from build123d import *

# Parameters (mm, degrees)
SKETCH1_R           = 3.25
SKETCH1_R_2         = 2.38125
SKETCH1_R_3         = 1.5875
SKETCH1_W           = 4
SKETCH1_H           = 4
BOSS_EXTRUDE1_DEPTH = 4


with BuildPart() as part:
    # Sketch1 → Boss-Extrude1 (new body)
    with BuildSketch(Plane(origin=(0, 0, 0), x_dir=(1, 0, 0), z_dir=(0, 1, 0))):
        with BuildLine():
            Line((-50.8, 14), (-36.8, 14))
            ThreePointArc((-36.8, 14), (-35.385786438, 13.414213562), (-34.8, 12))
            Line((-34.8, 12), (-34.8, 7.914556152))
            ThreePointArc((-34.8, 7.914556152), (-34.214213562, 6.500342589), (-32.8, 5.914556152))
            Line((-32.8, 5.914556152), (50.8, 5.914556152))
            ThreePointArc((50.8, 5.914556152), (56.714556152, 0), (50.8, -5.914556152))
            Line((50.8, -5.914556152), (-32.8, -5.914556152))
            ThreePointArc((-32.8, -5.914556152), (-34.214213562, -6.500342589), (-34.8, -7.914556152))
            Line((-34.8, -7.914556152), (-34.8, -12))
            ThreePointArc((-34.8, -12), (-35.385786438, -13.414213562), (-36.8, -14))
            Line((-36.8, -14), (-50.8, -14))
            Line((-50.8, -14), (-52.8, -14))
            ThreePointArc((-52.8, -14), (-66.8, 0), (-52.8, 14))
            Line((-52.8, 14), (-50.8, 14))
        make_face()
        with Locations(Location((-50.8, 0, 0), (0, 0, 270))):
            Circle(SKETCH1_R, mode=Mode.SUBTRACT)
        with Locations(Location((38.8, 0, 0), (0, 0, 270))):
            Circle(SKETCH1_R_2, mode=Mode.SUBTRACT)
        with Locations(Location((26.1, 0, 0), (0, 0, 270))):
            Circle(SKETCH1_R_3, mode=Mode.SUBTRACT)
        with BuildLine():
            Line((-57.252349378, 8.220116331), (-54.247145558, 5.214912511))
            ThreePointArc((-54.247145558, 5.214912511), (-54.247145558, 3.447145558), (-56.014912511, 3.447145558))
            Line((-56.014912511, 3.447145558), (-59.020116331, 6.452349378))
            ThreePointArc((-59.020116331, 6.452349378), (-59.020116331, 8.220116331), (-57.252349378, 8.220116331))
        make_face(mode=Mode.SUBTRACT)
        with BuildLine():
            Line((-42.579883669, 6.452349378), (-45.585087489, 3.447145558))
            ThreePointArc((-45.585087489, 3.447145558), (-47.352854442, 3.447145558), (-47.352854442, 5.214912511))
            Line((-47.352854442, 5.214912511), (-44.347650622, 8.220116331))
            ThreePointArc((-44.347650622, 8.220116331), (-42.579883669, 8.220116331), (-42.579883669, 6.452349378))
        make_face(mode=Mode.SUBTRACT)
        with BuildLine():
            Line((-44.347650622, -8.220116331), (-47.352854442, -5.214912511))
            ThreePointArc((-47.352854442, -5.214912511), (-47.352854442, -3.447145558), (-45.585087489, -3.447145558))
            Line((-45.585087489, -3.447145558), (-42.579883669, -6.452349378))
            ThreePointArc((-42.579883669, -6.452349378), (-42.579883669, -8.220116331), (-44.347650622, -8.220116331))
        make_face(mode=Mode.SUBTRACT)
        with BuildLine():
            Line((-59.020116331, -6.452349378), (-56.014912511, -3.447145558))
            ThreePointArc((-56.014912511, -3.447145558), (-54.247145558, -3.447145558), (-54.247145558, -5.214912511))
            Line((-54.247145558, -5.214912511), (-57.252349378, -8.220116331))
            ThreePointArc((-57.252349378, -8.220116331), (-59.020116331, -8.220116331), (-59.020116331, -6.452349378))
        make_face(mode=Mode.SUBTRACT)
        with Locations((49.8, 0)):
            Rectangle(SKETCH1_W, SKETCH1_H, mode=Mode.SUBTRACT)
        with Locations((-9.2, 0)):
            Rectangle(SKETCH1_W, SKETCH1_H, mode=Mode.SUBTRACT)
    extrude(amount=BOSS_EXTRUDE1_DEPTH)


solid = part.part
Read the model definition and answer for the solid it produces. Units are mm, in the model's axes. A direction names the side the tool comes from. Round coordinates to 2 decimals unless told otherwise and drop trailing zeros. Write each loop counter-clockwise with the first axis right and the second up, starting at its lowest first coordinate (ties: lowest second). Pieces come first, ordered by that corner, then holes.
Q1. The mould has two halves that part along Z. Classify faces 6 (the face through (-57.5, 1.97, -4.93)), 7 (the face through (-34.23, 1.972, -6.516)), 8 (the face through (56.713, 1.972, -0.13)): released by +Z, released by -Z, zero draft, split by the parting line, or undercut.
Values:
face 6: undercut
face 7: released by -Z
face 8: split by the parting line
Q2. Find section B-B on z = 0. Determine the outline of the cut face in (x, y).
Values:
outline: (-66.8, 0) - (-54.05, 0) - (-54.05, 4) - (-66.8, 4) - close; (-47.55, 0) - (-11.2, 0) - (-11.2, 4) - (-47.55, 4) - close; (-7.2, 0) - (24.51, 0) - (24.51, 4) - (-7.2, 4) - close; (27.69, 0) - (36.42, 0) - (36.42, 4) - (27.69, 4) - close; (41.18, 0) - (47.8, 0) - (47.8, 4) - (41.18, 4) - close; (51.8, 0) - (56.71, 0) - (56.71, 4) - (51.8, 4) - close
Q3. Find section D-D on y = 2.4. State how many separate pieces and enclosed holes the cut face has, and give its area (3 significant figures).
Values:
separate pieces: 1
enclosed holes: 9
area: 1,730 mm2
Q4. Straight lines are drawn through the part: line 1 (X direction, y = 2.35, z = 0); line 2 (Z direction, x = 51, y = 0.8); line 3 (X direction, y = 2.2, z = -0.75). For each, find the intervals that lie inside material, in ascending order.
Values:
line 1: x = -66.8 to -54.05, -47.55 to -11.2, -7.2 to 24.51, 27.69 to 36.42, 41.18 to 47.8, 51.8 to 56.71
line 2: z = -5.91 to -2, 2 to 5.91
line 3: x = -66.78 to -53.96, -47.64 to -11.2, -7.2 to 24.7, 27.5 to 36.54, 41.06 to 47.8, 51.8 to 56.67
Q5. Flat-ended cylindrical pins translate along their axes: P1, Ø1.2, axis at x = 14.5, y = 1.5, coming from the -Z side; P2, Ø2, axis at y = 1, z = -7.5, coming from the +X side; P3, Ø1.2, axis at x = 3.5, y = 3, coming from the +Z side. Find the tip coordinate at first contact, or state that the pin passes through.
Values:
P1: stops at z = -5.91
P2: stops at x = -34.21
P3: stops at z = 5.91
Q6. Find section A-A on x = 26.1. Determine the outline of the cut face in (y, z), and give its area (3 significant figures).
Values:
outline: (0, -5.91) - (4, -5.91) - (4, -1.59) - (0, -1.59) - close; (0, 1.59) - (4, 1.59) - (4, 5.91) - (0, 5.91) - close
area: 34.6 mm2
Q7. A tool of negligible diameter and unlimited length cuts with its end or side. For faces 1 (the face through (-18, 0, 0)), 2 (the face through (-18, 4, 0)), 3 (the face through (8, 2, -5.915)), 4 (the face through (-45.87, 1.97, -6.7)), 5 (the face through (-34.8, 2, 10)), from which of +Z, -Z, +X, -X, +Y, -Y can it reach the whole face along a straight path? Write none if from no direction.
Values:
face 1: +Z, -Z, +X, -X, -Y
face 2: +Z, -Z, +X, -X, +Y
face 3: -Z, +X, +Y, -Y
face 4: +Y, -Y
face 5: +Z, +X, +Y, -Y
Q8. Find section C-C on x = -50.8. Determine the outline of the cut face in (y, z), and give its area (3 significant figures).
Values:
outline: (0, -14) - (4, -14) - (4, -3.25) - (0, -3.25) - close; (0, 3.25) - (4, 3.25) - (4, 14) - (0, 14) - close
area: 86.0 mm2
